Work out the finished part from the listing and answer in its coordinate system (mm). A direction names the side the tool comes from. Coordinates: 2 decimals unless noted, no trailing zeros. Order: outer loops, then holes, each group sorted by start corner. A loop starts at its lowest first (then second) coordinate and runs counter-clockwise, first axis right, second up. Notation, with made-up numbers: M -3,-7.75 L 44,-7.75 A25 cw 44,5.25 Z; hole C 82.5,12.25 d2. An arc over 180 degrees is marked long. Use a Markdown table: item, result. Add a question column.
from build123d import *

# Parameters (mm, degrees)
SKETCH_W              = 18.5
SKETCH_H              = 18.5
SKETCH_R              = 8.15
PAD_DEPTH             = 4
SKETCH001_W           = 18.5
SKETCH001_H           = 18.5
PAD001_DEPTH          = 3
SKETCH002_R           = 9.25
SKETCH003_R           = 5.4
SKETCH005_R           = 5.4
PAD002_DEPTH          = 2
CHAMFER_SIZE          = 1.5
CHAMFER001_SIZE       = 1.5
POCKET_DEPTH          = 114.093887
POLARPATTERN_COUNT    = 4
SKETCH007_R           = 4.4
SKETCH008_R           = 5.4
SKETCH009_R           = 5.4
PAD003_DEPTH          = 13
SKETCH010_R           = 4.4
POCKET001_DEPTH       = 5
POCKET002_DEPTH       = 140.31233
POLARPATTERN001_COUNT = 3
POCKET003_DEPTH       = 18.501


with BuildPart() as part:
    # Sketch → Pad (new body)
    with BuildSketch(Plane.XY):
        Rectangle(SKETCH_W, SKETCH_H)
        Circle(SKETCH_R, mode=Mode.SUBTRACT)
    extrude(amount=PAD_DEPTH)

    # Sketch001 (on Face7 of Pad) → Pad001 (join)
    with BuildSketch(Plane.XY.offset(4)):
        Rectangle(SKETCH001_W, SKETCH001_H)
    extrude(amount=PAD001_DEPTH)

    # Sketch002 (on Face10 of Pad001) → AdditiveLoft section 0
    with BuildSketch(Plane.XY.offset(7)):
        Circle(SKETCH002_R)
    # Sketch003 (on Face10 of Pad001) → AdditiveLoft section 1
    with BuildSketch(Plane.XY.offset(38)):
        Circle(SKETCH003_R)
    loft()

    # Sketch005 (on Face17 of AdditiveLoft) → Pad002 (join)
    with BuildSketch(Plane.XY.offset(38)):
        Circle(SKETCH005_R)
    extrude(amount=PAD002_DEPTH)

    # Chamfer
    chamfer_edges = [part.edges().sort_by_distance(p)[0] for p in [
        (-9.25, -9.25, 5.5),
        (-9.25, -9.25, 2),
        (9.25, -9.25, 5.5),
        (9.25, -9.25, 2),
        (9.25, 9.25, 2),
        (9.25, 9.25, 5.5),
        (-9.25, 9.25, 5.5),
        (-9.25, 9.25, 2),
    ]]
    chamfer(chamfer_edges, length=CHAMFER_SIZE)

    # Chamfer001
    chamfer001_edges = [part.edges().sort_by_distance(p)[0] for p in [
        (8.5, -8.5, 7),
        (-8.5, -8.5, 7),
        (-8.5, 8.5, 7),
        (8.5, 8.5, 7),
    ]]
    chamfer(chamfer001_edges, length=CHAMFER001_SIZE)

    # Sketch006 (on Face19 of Chamfer001) → Pocket (cut, through all)
    with BuildSketch(Plane.YZ.offset(9.25)):
        Polygon((0, 38), (-2.7, 7), (2.7, 7), align=None)
    pocket = extrude(amount=-POCKET_DEPTH, mode=Mode.SUBTRACT)

    # PolarPattern: Pocket ×4 about axis
    polarpattern_axis = Axis((0, 0, 0), (0, 0, 1))
    for i in range(1, POLARPATTERN_COUNT):
        add(pocket.rotate(polarpattern_axis, i * 360 / POLARPATTERN_COUNT), mode=Mode.SUBTRACT)

    # Sketch007 (on Face47 of PolarPattern) → AdditiveLoft001 section 0
    with BuildSketch(Plane.XY.offset(40)):
        Circle(SKETCH007_R)
    # Sketch008 → AdditiveLoft001 section 1
    with BuildSketch(Plane.XY.offset(42)):
        Circle(SKETCH008_R)
    loft()

    # Sketch009 (on Face56 of AdditiveLoft001) → Pad003 (join)
    with BuildSketch(Plane.XY.offset(42)):
        Circle(SKETCH009_R)
    extrude(amount=PAD003_DEPTH)

    # Sketch010 (on Face57 of Pad003) → Pocket001 (cut)
    with BuildSketch(Plane.XY.offset(55)):
        Circle(SKETCH010_R)
    extrude(amount=-POCKET001_DEPTH, mode=Mode.SUBTRACT)

    # Sketch011 (on Face26 of Pocket001) → Pocket002 (cut, through all)
    with BuildSketch(Plane.YZ.offset(9.25)):
        Polygon((-1.75, 55), (1.75, 55), (0.85, 50), (-0.85, 50), align=None)
    pocket002 = extrude(amount=-POCKET002_DEPTH, mode=Mode.SUBTRACT)

    # PolarPattern001: Pocket002 ×3 about axis
    polarpattern001_axis = Axis((0, 0, 0), (0, 0, 1))
    for i in range(1, POLARPATTERN001_COUNT):
        add(pocket002.rotate(polarpattern001_axis, i * 360 / POLARPATTERN001_COUNT), mode=Mode.SUBTRACT)

    # Sketch012 (on Face1 of PolarPattern001) → Pocket003 (cut, through all)
    with BuildSketch(Plane(origin=(0, 9.25, 0), x_dir=(-1, 0, 0), z_dir=(0, 1, 0))):
        Polygon((-3, 46.5), (-0.5, 46.5), (-0.5, 49), (0.5, 49), (0.5, 46.5), (3, 46.5), (3, 45.5), (0.5, 45.5), (0.5, 43), (-0.5, 43), (-0.5, 45.5), (-3, 45.5), align=None)
    extrude(amount=-POCKET003_DEPTH, mode=Mode.SUBTRACT)


solid = part.part
(1) A cutting plane is placed at A-A on z = 14.5. Write down the section's boundary in (x, y), plus the area to 3 significant figures.
(2) Given P1, Ø3, axis at y = 0, z = 47.5, coming from the -X side; P2, Ø3, axis at x = -1.5, z = 43, coming from the +Y side; P3, Ø5, axis at x = 4.5, z = 27.5, coming from the -Y side; P4, Ø1.5, axis at x = 6.5, z = 37, coming from the -Y side, each flat-ended and moving along its own axis, determine where each tip first touches the part or whether it passes through.
(3) Which of the six approach directions +Z, -Z, +X, -X, +Y, -Y give full straight-line access (tool end or side, diameter ignored) to faces 1 (the flat face through (0, 0, 7)), 2 (the flat face through (-4.7, 1.3, 52.5)), 3 (the flat face through (0.5, 0, 48)), 4 (the flat face through (0, 0, 50))?
(4) A cutting plane is placed at C-C on z = 35. Write down the section's boundary in (x, y), plus the area to 3 significant figures.
(5) A cutting plane is placed at B-B on z = 51.5. Write down the section's boundary in (x, y) (3 decimals), plus the area to 3 significant figures.
(6) The mould has two halves that part along X. Classify faces 5 (the cylindrical face through (-5.395, 0.237, 48.409)), 6 (the flat face through (-4.3, -2.4, 55)), 7 (the flat face through (-1.37, -4.36, 22.28)), 8 (the flat face through (-7.88, 7.83, 6.41)): pulls with the +X half, pulls with the -X half, needs draft (parallel to the pull), parting line crosses it, or undercut.
(7) Straight lines are drawn through the part: line 1 (Y direction, x = 0, z = 2.75); line 2 (Z direction, x = 7.75, y = 0); line 3 (Z direction, x = -2.5, y = 8.75). For each, find the intervals that lie inside material, in ascending order.
From the geometry:
| question | item | result |
|---|---|---|
| 1 | outline | M -8.06,-2.05 A8.32 ccw -2.05,-8.06 L -2.05,-2.05 Z; M -8.06,2.05 L -2.05,2.05 L -2.05,8.06 A8.32 ccw Z; M 2.05,-8.06 A8.32 ccw 8.06,-2.05 L 2.05,-2.05 Z; M 2.05,2.05 L 8.06,2.05 A8.32 ccw 2.05,8.06 Z |
| 1 | area | 99.3 mm2 |
| 2 | P1 | stops at x = -5.4 |
| 2 | P2 | stops at y = 5.4 |
| 2 | P3 | stops at y = -6.46 |
| 2 | P4 | passes through |
| 3 | face 1 | none |
| 3 | face 2 | +Z, +X, -X |
| 3 | face 3 | +Y, -Y |
| 3 | face 4 | +Z |
| 4 | outline | M -5.77,-0.26 A5.77 ccw -0.26,-5.77 L -0.26,-0.26 Z; M -5.77,0.26 L -0.26,0.26 L -0.26,5.77 A5.77 ccw Z; M 0.26,-5.77 A5.77 ccw 5.77,-0.26 L 0.26,-0.26 Z; M 0.26,0.26 L 5.77,0.26 A5.77 ccw 0.26,5.77 Z |
| 4 | area | 92.9 mm2 |
| 5 | outline | M -5.283,-1.12 A5.4 ccw -3.611,-4.015 L -3.097,-3.125 A4.4 cw -4.255,-1.12 Z; M -5.283,1.12 L -4.255,1.12 A4.4 cw -3.097,3.125 L -3.611,4.015 A5.4 ccw Z; M -1.671,-5.135 A5.4 ccw 1.671,-5.135 L 1.158,-4.245 A4.4 cw -1.158,-4.245 Z; M -1.671,5.135 L -1.158,4.245 A4.4 cw 1.158,4.245 L 1.671,5.135 A5.4 ccw Z; M 3.097,-3.125 L 3.611,-4.015 A5.4 ccw 5.283,-1.12 L 4.255,-1.12 A4.4 cw Z; M 3.097,3.125 A4.4 cw 4.255,1.12 L 5.283,1.12 A5.4 ccw 3.611,4.015 Z |
| 5 | area | 17.2 mm2 |
| 6 | face 5 | parting line crosses it |
| 6 | face 6 | needs draft |
| 6 | face 7 | undercut |
| 6 | face 8 | pulls with the -X half |
| 7 | line 1 | y = -9.25 to -8.15, 8.15 to 9.25 |
| 7 | line 2 | z = 4 to 7 |
| 7 | line 3 | z = 0 to 7 |
